```python
from build123d import *

# Parameters (mm, degrees)
SKETCH1_W               = 390.8
SKETCH1_H               = 133.8
BOSS_EXTRUDE1_DEPTH     = 6
SKETCH2_W               = 370.8
SKETCH2_H               = 125.6
CUT_EXTRUDE1_DEPTH      = 4
BOSS_EXTRUDE3_DEPTH     = 390.8
SKETCH8_W               = 9.2
SKETCH8_H               = 4
CUT_EXTRUDE2_DEPTH      = 10
BOSS_EXTRUDE4_DEPTH     = 4
SKETCH11_W              = 15.2
SKETCH11_H              = 5.5
CUT_EXTRUDE3_DEPTH      = 1
CUT_EXTRUDE6_DEPTH      = 414.309625425
CUT_EXTRUDE6_DEPTH_BACK = 414.309625425
M2_CLEARANCE_HOLE1_D    = 2.4
CUT_EXTRUDE7_START      = -3
SKETCH13_R              = 2.5
CUT_EXTRUDE7_DEPTH      = 411.484592101
FILLET2_R               = 4
SKETCH15_R              = 5
CUT_EXTRUDE8_DEPTH      = 1
SKETCH16_W              = 11.5
SKETCH16_H              = 19.9
CUT_EXTRUDE9_DEPTH      = 6
FILLET1_R               = 4


with BuildPart() as part:
    # Sketch1 → Boss-Extrude1 (new body)
    with BuildSketch(Plane(origin=(0, 0, 0), x_dir=(1, 0, 0), z_dir=(0, 1, 0))):
        with Locations((195.4, 66.9)):
            Rectangle(SKETCH1_W, SKETCH1_H)
    extrude(amount=BOSS_EXTRUDE1_DEPTH)

    # Sketch2 → Cut-Extrude1 (cut)
    with BuildSketch(Plane(origin=(0, 6, 0), x_dir=(1, 0, 0), z_dir=(0, 1, 0))):
        with Locations((195.4, 68.4)):
            Rectangle(SKETCH2_W, SKETCH2_H)
    extrude(amount=-CUT_EXTRUDE1_DEPTH, mode=Mode.SUBTRACT)

    # Boss-Extrude3: read off the stored shape, not the designer's step
    # Boss-Extrude3 outline → Boss-Extrude3 (add)
    with BuildSketch(Plane.YZ):
        Polygon((-14.062946679, -133.8), (0, -133.8), (0, 0), align=None)
    extrude(amount=BOSS_EXTRUDE3_DEPTH)

    # Sketch8 → Cut-Extrude2 (cut)
    with BuildSketch(Plane(origin=(0, 0, -133.8), x_dir=(-1, 0, 0), z_dir=(0, 0, -1))):
        with Locations((-34.3, 4)):
            Rectangle(SKETCH8_W, SKETCH8_H)
    extrude(amount=-CUT_EXTRUDE2_DEPTH, mode=Mode.SUBTRACT)

    # Sketch10 → Boss-Extrude4 (add)
    with BuildSketch(Plane(origin=(0, 2, 0), x_dir=(1, 0, 0), z_dir=(0, 1, 0))):
        with BuildLine():
            Line((99.5, 5.6), (105.5, 5.6))
            ThreePointArc((105.5, 5.6), (102.5, 8.6), (99.5, 5.6))
        make_face()
        with BuildLine():
            ThreePointArc((290.5, 5.6), (287.5, 8.6), (284.5, 5.6))
            Line((284.5, 5.6), (290.5, 5.6))
        make_face()
        with BuildLine():
            ThreePointArc((284.5, 131.2), (287.5, 128.2), (290.5, 131.2))
            Line((290.5, 131.2), (284.5, 131.2))
        make_face()
        with BuildLine():
            ThreePointArc((192.4, 131.2), (195.4, 128.2), (198.4, 131.2))
            Line((198.4, 131.2), (192.4, 131.2))
        make_face()
        with BuildLine():
            Line((105.5, 131.2), (99.5, 131.2))
            ThreePointArc((99.5, 131.2), (102.5, 128.2), (105.5, 131.2))
        make_face()
    extrude(amount=BOSS_EXTRUDE4_DEPTH)

    # Sketch11 → Cut-Extrude3 (cut)
    with BuildSketch(Plane(origin=(0, 0, -133.8), x_dir=(-1, 0, 0), z_dir=(0, 0, -1))):
        with Locations((-34.3, 3.25)):
            Rectangle(SKETCH11_W, SKETCH11_H)
    extrude(amount=-CUT_EXTRUDE3_DEPTH, mode=Mode.SUBTRACT)

    # Sketch12 → Cut-Extrude6 (cut, two sides: drawn at the far end of the back side and taken through both)
    with BuildSketch(Plane.ZY.offset(-CUT_EXTRUDE6_DEPTH_BACK)):
        Polygon((-133.8, -14.062946679), (-118.975297196, -12.504807627), (-133.8, -0.5), align=None)
    extrude(amount=CUT_EXTRUDE6_DEPTH + CUT_EXTRUDE6_DEPTH_BACK, mode=Mode.SUBTRACT)

    # M2 Clearance Hole1 (through all)
    with Locations(Plane(origin=(102.5, 6, -5.6), x_dir=(0, 0, 1), z_dir=(0, 1, 0))):
        with Locations((0, 0), (-39.4, -97.2), (-83.2, -97.2), (-125.6, 0), (-125.6, 92.9), (-125.6, 185), (-83.2, 283), (-39.4, 283), (0, 185)):
            Hole(M2_CLEARANCE_HOLE1_D / 2)

    # Sketch13 → Cut-Extrude7 (cut, through all)
    with BuildSketch(Plane(origin=(0, 6, 0), x_dir=(1, 0, 0), z_dir=(0, 1, 0)).offset(CUT_EXTRUDE7_START)):
        with Locations(Location((5.3, 45, 0), (0, 0, 270))):
            Circle(SKETCH13_R)
        with Locations(Location((5.3, 88.8, 0), (0, 0, 270))):
            Circle(SKETCH13_R)
        with Locations(Location((102.5, 5.6, 0), (0, 0, 270))):
            Circle(SKETCH13_R)
        with Locations(Location((287.5, 5.6, 0), (0, 0, 270))):
            Circle(SKETCH13_R)
        with Locations(Location((385.5, 45, 0), (0, 0, 270))):
            Circle(SKETCH13_R)
        with Locations(Location((385.5, 88.8, 0), (0, 0, 270))):
            Circle(SKETCH13_R)
        with Locations(Location((287.5, 131.2, 0), (0, 0, 270))):
            Circle(SKETCH13_R)
        with Locations(Location((195.4, 131.2, 0), (0, 0, 270))):
            Circle(SKETCH13_R)
        with Locations(Location((102.5, 131.2, 0), (0, 0, 270))):
            Circle(SKETCH13_R)
    extrude(amount=-CUT_EXTRUDE7_DEPTH, mode=Mode.SUBTRACT)

    # Fillet2
    # the kernel refuses this fillet: 4 mm, written as the material it adds along each edge
    with BuildSketch(Plane(origin=(41.9, 0.5, -132.8), x_dir=(-1, 0, 0), z_dir=(0, 1, 0))) as fillet2_piece_1:
        with BuildLine():
            CenterArc((2.645751311, -4), FILLET2_R, 90, 41.409622109)
            Line((0, -1), (0, 0))
            Line((0, 0), (2.645751311, 0))
        make_face()
    extrude(amount=5.5)
    with BuildSketch(Plane(origin=(26.7, 6, -132.8), x_dir=(0, 0, -1), z_dir=(0, -1, 0))) as fillet2_piece_2:
        with BuildLine():
            CenterArc((4, 2.645751311), FILLET2_R, 180, 41.409622109)
            Line((0, 2.645751311), (0, 0))
            Line((0, 0), (1, 0))
        make_face()
    extrude(amount=5.5)

    # Sketch15 → Cut-Extrude8 (cut)
    with BuildSketch(Plane(origin=(0, 0, 0), x_dir=(1, 0, 0), z_dir=(0, -0.9945218953682742, 0.10452846326764666))):
        with Locations(Location((15, -109.630646394, 0), (0, 0, 270))):
            Circle(SKETCH15_R)
        with Locations(Location((375.8, -109.630646394, 0), (0, 0, 270))):
            Circle(SKETCH15_R)
        with Locations(Location((15, -10, 0), (0, 0, 270))):
            Circle(SKETCH15_R)
        with Locations(Location((375.8, -10, 0), (0, 0, 270))):
            Circle(SKETCH15_R)
    extrude(amount=-CUT_EXTRUDE8_DEPTH, mode=Mode.SUBTRACT)

    # Sketch16 → Cut-Extrude9 (cut)
    with BuildSketch(Plane(origin=(0, 6, 0), x_dir=(1, 0, 0), z_dir=(0, 1, 0))):
        with Locations((15.75, 47.15)):
            Rectangle(SKETCH16_W, SKETCH16_H)
    extrude(amount=-CUT_EXTRUDE9_DEPTH, mode=Mode.SUBTRACT)

    # Fillet1
    fillet1_edges = [part.edges().sort_by_distance(p)[0] for p in [
        (10, 4, -5.6),
        (10, 4, -131.2),
        (380.8, 4, -131.2),
        (380.8, 4, -5.6),
        (10, 1, -37.2),
        (10, 1, -57.1),
        (21.5, 1, -57.1),
        (21.5, 1, -37.2),
        (99.5, 4, -131.2),
        (105.5, 4, -131.2),
        (192.4, 4, -131.2),
        (198.4, 4, -131.2),
        (284.5, 4, -131.2),
        (290.5, 4, -131.2),
        (290.5, 4, -5.6),
        (284.5, 4, -5.6),
        (105.5, 4, -5.6),
        (99.5, 4, -5.6),
    ]]
    fillet(fillet1_edges, radius=FILLET1_R)


solid = part.part
```
Design review of the part built by this model. Coordinates are the model's own, in mm. A direction names the side the tool comes from. Round coordinates to 2 decimals unless told otherwise and drop trailing zeros. Write each loop counter-clockwise with the first axis right and the second up, starting at its lowest first coordinate (ties: lowest second). Pieces come first, ordered by that corner, then holes.
Item 1: For probe 1 along X at (y, z) = (-2.75, -45); probe 2 along X at (y, z) = (0.5, -5.6); probe 3 along Z at (x, y) = (385.5, 5), list the stretches that pass through material, from the lowest coordinate up.
Item 2: We need section B-B on z = -22.5. Write out the cut boundary in (x, y), and give its area (3 significant figures).
Item 3: We need section A-A on x = 277.5. Write out the cut boundary in (y, z).
Item 4: The part is to be moulded in two halves that separate along X. For faces 3 (the flat face through (390.8, -1, -81)), 4 (the cylindrical face through (10.12, -0.44, -8.92)), 5 (the flat face through (198, 2, -70)), 6 (the flat face through (0, -1, -81)), say which applies: +X half, -X half, draft (parallel to the pull), parting line (faces both ways), or undercut.
Item 5: Clearance check with flat-ended pins moving along their axes: pin 1 Ø3 at (x, z) = (195.4, -131.2) entering from -Y; pin 2 Ø5.5 at (x, z) = (6.5, -88.5) entering from -Y; pin 3 Ø3 at (x, z) = (64.5, -117.5) entering from +Y. State where each tip first meets the part, or that it passes through.
Item 6: For faces 1 (the flat face through (192.664, -6.165, -58.655)), 2 (the flat face through (16, 0, -47)), list the 3-axis set-ups (+Z, -Z, +X, -X, +Y, -Y) from which the entire face can be reached by the end or side of a thin tool; tool diameter is ignored.
Returned:
1. probe 1: x = 0 to 2.8, 7.8 to 383, 388 to 390.8
1. probe 2: x = 0 to 100, 105 to 285, 290 to 390.8
1. probe 3: z = -133.8 to -90, -87.6 to -46.2, -43.8 to 0
2. outline: (0, -2.36) - (390.8, -2.36) - (390.8, 6) - (380.8, 6) - (380.8, 2) - (10, 2) - (10, 6) - (0, 6) - close
2. area: 1,790 mm2
3. outline: (-12.5, -118.98) - (-0.5, -133.8) - (6, -133.8) - (6, -131.2) - (2, -131.2) - (2, -5.6) - (6, -5.6) - (6, 0) - (0, 0) - close
4. face 3: +X half
4. face 4: undercut
4. face 5: undercut
4. face 6: -X half
5. pin 1: stops at y = 3
5. pin 2: stops at y = -9.59
5. pin 3: stops at y = 2
6. face 1: +Z, +X, -X, -Y
6. face 2: +Y
